Job drawing, mm, ordinate dimensions from the low corner. One solid piece. A direction names the side the tool comes from. Round coordinates to 2 decimals unless told otherwise and drop trailing zeros. Loops run counter-clockwise (first coordinate to the right, second up) from the corner with the lowest first, then second, coordinate; pieces in that order, holes last.
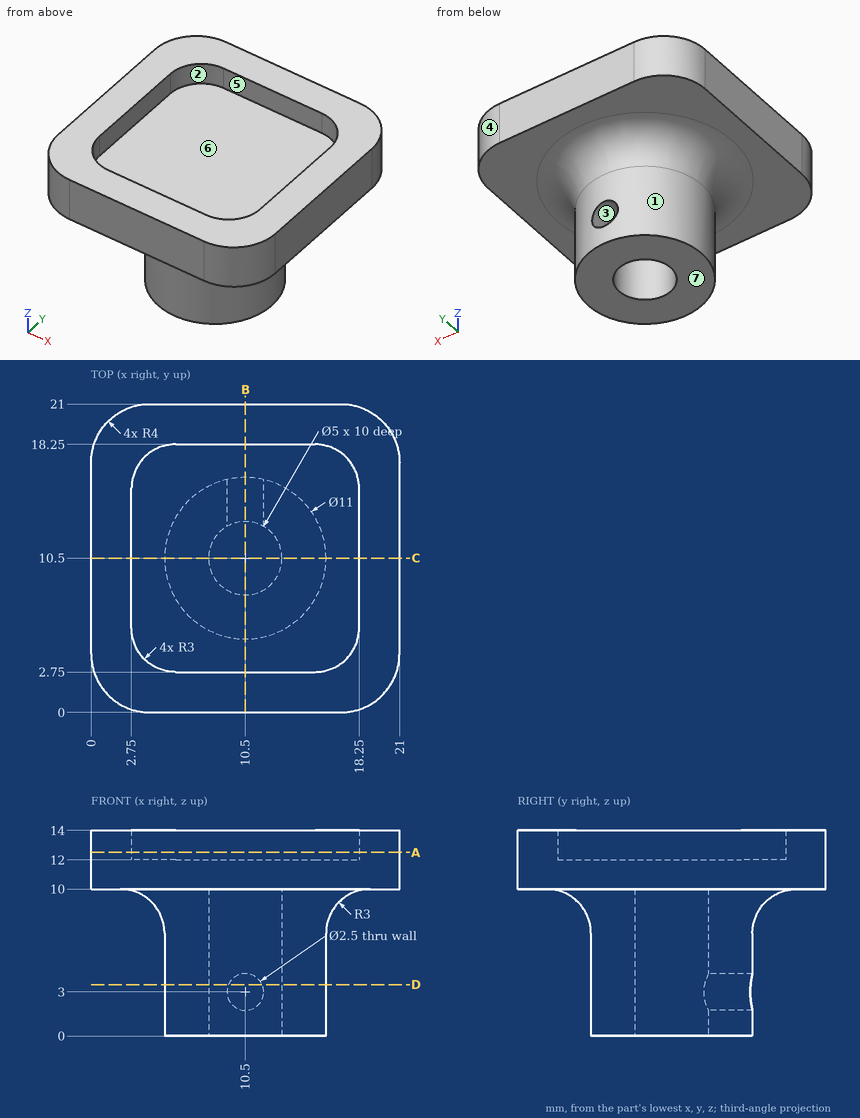
1) Mould opens along Y. For the marked faces 4, 5, 6 and 7 say: released by +Y, released by -Y, zero draft, split by the parting line, or undercut.
Values:
face 4: released by +Y
face 5: undercut
face 6: undercut
face 7: zero draft
2) Wall check: line 1 along Z through (x, y) = (10.5, 15.15); line 2 along Y through (x, z) = (10.5, 6); line 3 along Z through (x, y) = (6.5, 12.5). Give the ranges that are in metal, low to high.
Values:
line 1: z = 0 to 1.75, 4.25 to 12
line 2: y = 5 to 8, 13 to 16
line 3: z = 0 to 12
3) Tool access for the marked faces 1, 2 and 3: list every direction of +Z, -Z, +X, -X, +Y, -Y with a clear straight run to the whole face (end or side of a thin tool).
Values:
face 1: -Z
face 2: +Z
face 3: +Y
4) Drop flat-ended pins along their axis: pin 1 Ø8 at (y, z) = (14, 3) entering from +X; pin 2 Ø1.5 at (x, y) = (9.5, 11) entering from -Z; pin 3 Ø2 at (x, z) = (10.5, 3) entering from -Y. Give the stop position or say it passes through.
Values:
pin 1: stops at x = 16
pin 2: stops at z = 10
pin 3: stops at y = 5
5) Slice it at A-A, the plane z = 12.5. Give the cut face in (x, y), then the cut area to 3 significant figures.
Values:
outline: (0, 4) arc R4 ccw to (4, 0) - (17, 0) arc R4 ccw to (21, 4) - (21, 17) arc R4 ccw to (17, 21) - (4, 21) arc R4 ccw to (0, 17) - close; hole (2.75, 5.75) arc R3 ccw to (5.75, 2.75) - (15.25, 2.75) arc R3 ccw to (18.25, 5.75) - (18.25, 15.25) arc R3 ccw to (15.25, 18.25) - (5.75, 18.25) arc R3 ccw to (2.75, 15.25) - close
area: 195 mm2
6) Slice it at B-B, the plane x = 10.5. Give the cut face in (y, z).
Values:
outline: (0, 10) - (2, 10) arc R3 cw to (5, 7) - (5, 0) - (8, 0) - (8, 10) - (13, 10) - (13, 4.25) - (16, 4.25) - (16, 7) arc R3 cw to (19, 10) - (21, 10) - (21, 14) - (18.25, 14) - (18.25, 12) - (2.75, 12) - (2.75, 14) - (0, 14) - close; (13, 0) - (16, 0) - (16, 1.75) - (13, 1.75) - close
7) Slice it at C-C, the plane y = 10.5. Give the cut face in (x, z), then the cut area to 3 significant figures.
Values:
outline: (0, 10) - (2, 10) arc R3 cw to (5, 7) - (5, 0) - (8, 0) - (8, 10) - (13, 10) - (13, 0) - (16, 0) - (16, 7) arc R3 cw to (19, 10) - (21, 10) - (21, 14) - (18.25, 14) - (18.25, 12) - (2.75, 12) - (2.75, 14) - (0, 14) - close
area: 117 mm2
8) Slice it at D-D, the plane z = 3.5. Give the cut face in (x, y), then the cut area to 3 significant figures.
Values:
outline: (9.35, 12.72) - (9.35, 15.88) arc R5.5 ccw (long way) to (11.65, 15.88) - (11.65, 12.72) arc R2.5 cw (long way) to start
area: 68.4 mm2
